Work out the finished part from the listing and answer in its coordinate system (mm). A direction names the side the tool comes from. Coordinates: 2 decimals unless noted, no trailing zeros. Write each loop counter-clockwise with the first axis right and the second up, starting at its lowest first coordinate (ties: lowest second). Pieces come first, ordered by that corner, then holes. Notation, with made-up numbers: M -23,10 L 8,10 A23 cw 8,22 Z; hole C 57.25,-38.5 d7. An arc over 180 degrees is marked long. Answer as CSV lines item,"result". Start each with the question number.
(1) A cutting plane is placed at D-D on y = 10. Give the vertices of the cut face in (x, z), then the cut area to 3 significant figures.
(2) For faces 1 (the flat face through (80, 26.5, 2)), 2 (the flat face through (74.919, 16, 3)), 3 (the flat face through (45, 24.283, 2)), 4 (the flat face through (0, 17, 2)), determine the directions among +Z, -Z, +X, -X, +Y, -Y from which every point of the face is accessible in a straight line to the end or side of a thin tool.
(3) A cutting plane is placed at B-B on y = 28. Give the vertices of the cut face in (x, z), then the cut area to 3 significant figures.
(4) The mould has two halves that part along X. Classify faces 5 (the flat face through (45, 8.283, 2)), 6 (the flat face through (76.5, 16, 2)), 7 (the flat face through (59, 17, 0)): released by +X, released by -X, zero draft, split by the parting line, or undercut.
(5) A cutting plane is placed at C-C on z = 2.7. Count the separate pieces of the cut face and the enclosed holes in it, then the cut area to 3 significant figures.
(6) Flat-ended cylindrical pins translate along their axes: P1, Ø1.2, axis at y = 15, z = 2.5, coming from the +X side; P2, Ø4, axis at x = 17, y = 27.5, coming from the +Z side. Find the tip coordinate at first contact, or state that the pin passes through.
(7) A cutting plane is placed at A-A on x = 55. Give the vertices of the cut face in (y, z), then the cut area to 3 significant figures.
(8) Find the intervals of material crossed by L1, parallel to X at y = 15, z = 1.75; L2, parallel to X at y = 13.5, z = 3.2; L3, parallel to Y at x = 44, z = 0.6, in increasing order. Write a range as [from, to].
from build123d import *

# Parameters (mm, degrees)
SKETCH001_W  = 17
SKETCH001_H  = 16
PAD001_DEPTH = 2
SKETCH005_W  = 2.5
SKETCH005_H  = 18
PAD005_DEPTH = 4
SKETCH_W     = 26
SKETCH_H     = 25
SKETCH_W_2   = 25
SKETCH_H_2   = 16
PAD_DEPTH    = 4


with BuildPart() as cuerpo001:
    # Sketch001 → Pad001 (new body)
    with BuildSketch(Plane.XY):
        with Locations((66.419464, 16.283001)):
            Rectangle(SKETCH001_W, SKETCH001_H)
    extrude(amount=PAD001_DEPTH)


with BuildPart() as cuerpo001_1:
    # Body001 placement: moved
    add(cuerpo001.part.moved(Location((0, 0, 2))))


with BuildPart() as cuerpo005:
    # Sketch005 → Pad005 (new body)
    with BuildSketch(Plane.XY):
        with Locations((59.25, 16.380761)):
            Rectangle(SKETCH005_W, SKETCH005_H)
    extrude(amount=PAD005_DEPTH)


with BuildPart() as cuerpo:
    # Sketch → Pad (new body)
    with BuildSketch(Plane.XY):
        Polygon((0, 33.015301), (0, 0.015301), (83, 0.015301), (83, 6.5), (76.500001, 6.5), (76.500001, 26.5), (83, 26.5), (83, 33.015301), align=None)
        with Locations((16.5, 16.282843)):
            Rectangle(SKETCH_W, SKETCH_H, mode=Mode.SUBTRACT)
        with Locations((45.5, 16.282843)):
            Rectangle(SKETCH_W_2, SKETCH_H_2, mode=Mode.SUBTRACT)
    extrude(amount=PAD_DEPTH)

    # Boolean: cut Cuerpo001
    add(cuerpo001_1.part, mode=Mode.SUBTRACT)

    # Boolean001: union Cuerpo005
    add(cuerpo005.part)


solid = cuerpo.part
Here are the results:
1,outline,"M 0,0 L 3.5,0 L 3.5,4 L 0,4 Z; M 29.5,0 L 33,0 L 33,4 L 29.5,4 Z; M 58,0 L 76.5,0 L 76.5,4 L 74.92,4 L 74.92,2 L 60.5,2 L 60.5,4 L 58,4 Z"
1,area,"73.2 mm^2"
2,face 1,"+Z, -Z, +X"
2,face 2,"+Z"
2,face 3,"+Z, -Z"
2,face 4,"+Z, -Z, -X, +Y, -Y"
3,outline,"M 0,0 L 3.5,0 L 3.5,4 L 0,4 Z; M 29.5,0 L 83,0 L 83,4 L 29.5,4 Z"
3,area,"228 mm^2"
4,face 5,"undercut"
4,face 6,"released by +X"
4,face 7,"zero draft"
5,separate pieces,"1"
5,enclosed holes,"3"
5,area,"1,330 mm^2"
6,P1,"stops at x = 76.5"
6,P2,"stops at z = 4"
7,outline,"M 0.02,0 L 8.28,0 L 8.28,4 L 0.02,4 Z; M 24.28,0 L 33.02,0 L 33.02,4 L 24.28,4 Z"
7,area,"68.0 mm^2"
8,L1,"x = [0, 3.5], [29.5, 33], [58, 76.5]"
8,L2,"x = [0, 3.5], [29.5, 33], [58, 60.5], [74.92, 76.5]"
8,L3,"y = [0.02, 8.28], [24.28, 33.02]"
